For this review, take the finished solid that the model builds, in its own axes (mm). Face numbers are marked on the shaded views. A direction names the side the tool comes from. Round coordinates to 2 decimals unless told otherwise and drop trailing zeros. Order: outer loops, then holes, each group sorted by start corner. A loop starts at its lowest first (then second) coordinate and runs counter-clockwise, first axis right, second up.
from build123d import *
from OCP.BRepFilletAPI import BRepFilletAPI_MakeChamfer

# Parameters (mm, degrees)
SKETCH1_W           = 10.16
SKETCH1_H           = 25.4
BOSS_EXTRUDE1_DEPTH = 10.16
CHAMFER1_SIZE       = 5.08
CHAMFER1_SIZE2      = 3.557054294
CHAMFER6_SIZE       = 22.86
CHAMFER6_SIZE2      = 3.212763481
CHAMFER7_SIZE       = 22.86
CHAMFER7_SIZE2      = 3.212763481
CHAMFER10_SIZE2     = 1.466469684
CHAMFER10_SIZE      = 2.54
CHAMFER11_SIZE2     = 2.54
CHAMFER11_SIZE      = 1.466469684
BOSS_EXTRUDE2_DEPTH = 11.43
CHAMFER12_SIZE      = 20.32
CHAMFER12_SIZE_2    = 1.777769643
CHAMFER13_SIZE      = 1.27
CHAMFER13_SIZE2     = 0.703075315
CHAMFER13_SIZE2_2   = 0.738460687
CHAMFER14_SIZE      = 1.27
CHAMFER14_SIZE2     = 0.703075315
CHAMFER14_SIZE2_2   = 0.738460687
CHAMFER15_SIZE      = 29.032332849
CHAMFER15_SIZE_2    = 2.54
SCALE1_SCALE        = 1.5
BOSS_EXTRUDE4_DEPTH = 0.254


# Some blends are built 0.0001 mm under size
with BuildPart() as part:
    # Sketch1 → Boss-Extrude1 (new body)
    with BuildSketch(Plane.XY):
        with Locations((5.08, 12.7)):
            Rectangle(SKETCH1_W, SKETCH1_H)
    extrude(amount=BOSS_EXTRUDE1_DEPTH)

    # Chamfer1
    chamfer1_edges = [part.edges().sort_by_distance(p)[0] for p in [
        (5.08, 25.4, 10.16),
    ]]
    chamfer1_side = [part.faces().sort_by_distance(p)[0] for p in [
        (5.08, 12.7, 10.16),
    ]]
    chamfer(chamfer1_edges, length=CHAMFER1_SIZE, length2=CHAMFER1_SIZE2, reference=chamfer1_side[0])

    # Chamfer6
    chamfer6_edges = [part.edges().sort_by_distance(p)[0] for p in [
        (0, 0, 5.08),
    ]]
    chamfer6_side = [part.faces().sort_by_distance(p)[0] for p in [
        (0, 12.300671821, 4.93871201),
    ]]
    chamfer(chamfer6_edges, length=CHAMFER6_SIZE, length2=CHAMFER6_SIZE2, reference=chamfer6_side[0])

    # Chamfer7
    chamfer7_edges = [part.edges().sort_by_distance(p)[0] for p in [
        (10.16, 0, 5.08),
    ]]
    chamfer7_side = [part.faces().sort_by_distance(p)[0] for p in [
        (10.16, 12.300671821, 4.93871201),
    ]]
    chamfer(chamfer7_edges, length=CHAMFER7_SIZE, length2=CHAMFER7_SIZE2, reference=chamfer7_side[0])

    # Chamfer10
    chamfer10_edges = [part.edges().sort_by_distance(p)[0] for p in [
        (0, 25.4, 3.301472853),
    ]]
    chamfer10_side = [part.faces().sort_by_distance(p)[0] for p in [
        (0, 25.370670606, 3.301472853),
    ]]
    chamfer(chamfer10_edges, length=CHAMFER10_SIZE - 0.0001, length2=CHAMFER10_SIZE2 - 0.0001, reference=chamfer10_side[0])  # a hair under: the kernel refuses the full size

    # Chamfer11
    chamfer11_edges = [part.edges().sort_by_distance(p)[0] for p in [
        (10.16, 25.4, 3.301472853),
    ]]
    chamfer11_side = [part.faces().sort_by_distance(p)[0] for p in [
        (10.130670606, 25.4, 3.301472853),
    ]]
    chamfer(chamfer11_edges, length=CHAMFER11_SIZE - 0.0001, length2=CHAMFER11_SIZE2 - 0.0001, reference=chamfer11_side[0])  # a hair under: the kernel refuses the full size

    # Sketch2 → Boss-Extrude2 (add)
    with BuildSketch(Plane(origin=(0, 0, 0), x_dir=(-1, 0, 0), z_dir=(0, 0, -1))):
        Polygon((-5.08, 22.86), (-3.81, 22.86), (-3.81, 12.7), (-5.08, 12.7), (-6.35, 12.7), (-6.35, 22.86), align=None)
    extrude(amount=-BOSS_EXTRUDE2_DEPTH)

    # Chamfer12
    # the kernel refuses this chamfer: 20.32, 1.777769643 mm, written as the material it takes off along each edge
    with BuildSketch(Plane(origin=(-49.611801021, 0, 10.16), x_dir=(0, 0.9999943799678764, 0.003352615794033212), z_dir=(1, 0, 0))) as chamfer12_piece_1_section:
        Polygon((CHAMFER12_SIZE * 0.999994379968, -CHAMFER12_SIZE * 0.00335261579403), (-CHAMFER12_SIZE_2 * 0.00335261579374, -CHAMFER12_SIZE_2 * 0.999994379882), (0, 0), align=None)
    chamfer12_piece_1 = extrude(amount=109.383602042, mode=Mode.PRIVATE)
    chamfer12_piece_1 = split(chamfer12_piece_1, bisect_by=Plane(origin=(3.81, 16.274065634, 10.201831789), z_dir=(-1, 0, 0)), keep=Keep.TOP, mode=Mode.PRIVATE)
    chamfer12_piece_1 = split(chamfer12_piece_1, bisect_by=Plane(origin=(-22.90090051, 12.7, 10.201831789), z_dir=(0, 1, 0)), keep=Keep.TOP, mode=Mode.PRIVATE)
    add(chamfer12_piece_1, mode=Mode.SUBTRACT)
    with BuildSketch(Plane(origin=(-49.611801021, 0, 10.16), x_dir=(0, 0.9999943799678764, 0.003352615794033212), z_dir=(1, 0, 0))) as chamfer12_piece_2_section:
        Polygon((CHAMFER12_SIZE * 0.999994379968, -CHAMFER12_SIZE * 0.00335261579403), (-CHAMFER12_SIZE_2 * 0.00335261579374, -CHAMFER12_SIZE_2 * 0.999994379882), (0, 0), align=None)
    chamfer12_piece_2 = extrude(amount=109.383602042, mode=Mode.PRIVATE)
    chamfer12_piece_2 = split(chamfer12_piece_2, bisect_by=Plane(origin=(3.81, 5.349834898, 9.691469829), z_dir=(-1, 0, 0)), keep=Keep.TOP, mode=Mode.PRIVATE)
    chamfer12_piece_2 = split(chamfer12_piece_2, bisect_by=Plane(origin=(-22.90090051, 12.7, 9.691469829), z_dir=(0, -1, 0)), keep=Keep.TOP, mode=Mode.PRIVATE)
    add(chamfer12_piece_2, mode=Mode.SUBTRACT)
    with BuildSketch(Plane(origin=(-49.611801021, 0, 10.16), x_dir=(0, 0.9999943799678764, 0.003352615794033212), z_dir=(1, 0, 0))) as chamfer12_piece_3_section:
        Polygon((CHAMFER12_SIZE * 0.999994379968, -CHAMFER12_SIZE * 0.00335261579403), (-CHAMFER12_SIZE_2 * 0.00335261579374, -CHAMFER12_SIZE_2 * 0.999994379882), (0, 0), align=None)
    chamfer12_piece_3 = extrude(amount=109.383602042, mode=Mode.PRIVATE)
    chamfer12_piece_3 = split(chamfer12_piece_3, bisect_by=Plane(origin=(3.81, 5.349834898, 9.691469829), z_dir=(1, 0, 0)), keep=Keep.TOP, mode=Mode.PRIVATE)
    chamfer12_piece_3 = split(chamfer12_piece_3, bisect_by=Plane(origin=(5.08, 12.7, 9.691469829), z_dir=(0, -1, 0)), keep=Keep.TOP, mode=Mode.PRIVATE)
    chamfer12_piece_3 = split(chamfer12_piece_3, bisect_by=Plane(origin=(6.35, 5.349834898, 9.691469829), z_dir=(-1, 0, 0)), keep=Keep.TOP, mode=Mode.PRIVATE)
    add(chamfer12_piece_3, mode=Mode.SUBTRACT)
    with BuildSketch(Plane(origin=(-49.611801021, 0, 10.16), x_dir=(0, 0.9999943799678764, 0.003352615794033212), z_dir=(1, 0, 0))) as chamfer12_piece_4_section:
        Polygon((CHAMFER12_SIZE * 0.999994379968, -CHAMFER12_SIZE * 0.00335261579403), (-CHAMFER12_SIZE_2 * 0.00335261579374, -CHAMFER12_SIZE_2 * 0.999994379882), (0, 0), align=None)
    chamfer12_piece_4 = extrude(amount=109.383602042, mode=Mode.PRIVATE)
    chamfer12_piece_4 = split(chamfer12_piece_4, bisect_by=Plane(origin=(33.06090051, 12.7, 10.201831789), z_dir=(0, 1, 0)), keep=Keep.TOP, mode=Mode.PRIVATE)
    chamfer12_piece_4 = split(chamfer12_piece_4, bisect_by=Plane(origin=(6.35, 16.274065634, 10.201831789), z_dir=(1, 0, 0)), keep=Keep.TOP, mode=Mode.PRIVATE)
    add(chamfer12_piece_4, mode=Mode.SUBTRACT)
    with BuildSketch(Plane(origin=(-49.611801021, 0, 10.16), x_dir=(0, 0.9999943799678764, 0.003352615794033212), z_dir=(1, 0, 0))) as chamfer12_piece_5_section:
        Polygon((CHAMFER12_SIZE * 0.999994379968, -CHAMFER12_SIZE * 0.00335261579403), (-CHAMFER12_SIZE_2 * 0.00335261579374, -CHAMFER12_SIZE_2 * 0.999994379882), (0, 0), align=None)
    chamfer12_piece_5 = extrude(amount=109.383602042, mode=Mode.PRIVATE)
    chamfer12_piece_5 = split(chamfer12_piece_5, bisect_by=Plane(origin=(33.06090051, 12.7, 9.691469829), z_dir=(0, -1, 0)), keep=Keep.TOP, mode=Mode.PRIVATE)
    chamfer12_piece_5 = split(chamfer12_piece_5, bisect_by=Plane(origin=(6.35, 5.349834898, 9.691469829), z_dir=(1, 0, 0)), keep=Keep.TOP, mode=Mode.PRIVATE)
    add(chamfer12_piece_5, mode=Mode.SUBTRACT)

    # Chamfer13: one chamfer whose edges measure the first distance from different faces: ONE call of the kernel's chamfer builder (chamfer() names one face for all edges)
    chamfer13_edges_1 = [part.edges().sort_by_distance(p)[0] for p in [
        (0.17848686, 21.59, 9.270736426),
    ]]
    chamfer13_side_1 = [part.faces().sort_by_distance(p)[0] for p in [
        (5.08, 22.944432903, 8.322352298),
    ]]
    chamfer13_edges_2 = [part.edges().sort_by_distance(p)[0] for p in [
        (1.784868601, 10.16, 9.271115179),
    ]]
    chamfer13_side_2 = [part.faces().sort_by_distance(p)[0] for p in [
        (1.566458565, 11.714068156, 4.649741863),
    ]]
    chamfer13 = BRepFilletAPI_MakeChamfer(part.part.solid().wrapped)
    for e in chamfer13_edges_1:
        chamfer13.Add(CHAMFER13_SIZE, CHAMFER13_SIZE2, e.wrapped, chamfer13_side_1[0].wrapped)  # the first distance lies on this face
    for e in chamfer13_edges_2:
        chamfer13.Add(CHAMFER13_SIZE, CHAMFER13_SIZE2_2, e.wrapped, chamfer13_side_2[0].wrapped)  # the first distance lies on this face
    add(Compound.cast(chamfer13.Shape()), mode=Mode.REPLACE)

    # Chamfer14: one chamfer whose edges measure the first distance from different faces: ONE call of the kernel's chamfer builder (chamfer() names one face for all edges)
    chamfer14_edges_1 = [part.edges().sort_by_distance(p)[0] for p in [
        (9.98151314, 21.59, 9.270736426),
    ]]
    chamfer14_side_1 = [part.faces().sort_by_distance(p)[0] for p in [
        (8.593541435, 11.714068156, 4.649741863),
    ]]
    chamfer14_edges_2 = [part.edges().sort_by_distance(p)[0] for p in [
        (8.375131399, 10.16, 9.271115179),
    ]]
    chamfer14_side_2 = [part.faces().sort_by_distance(p)[0] for p in [
        (5.530551527, 10.889375046, 9.334927227),
    ]]
    chamfer14 = BRepFilletAPI_MakeChamfer(part.part.solid().wrapped)
    for e in chamfer14_edges_1:
        chamfer14.Add(CHAMFER14_SIZE, CHAMFER14_SIZE2, e.wrapped, chamfer14_side_1[0].wrapped)  # the first distance lies on this face
    for e in chamfer14_edges_2:
        chamfer14.Add(CHAMFER14_SIZE, CHAMFER14_SIZE2_2, e.wrapped, chamfer14_side_2[0].wrapped)  # the first distance lies on this face
    add(Compound.cast(chamfer14.Shape()), mode=Mode.REPLACE)

    # Chamfer15
    # the kernel refuses this chamfer: 29.032332849, 2.54 mm, written as the material it takes off along each edge
    with BuildSketch(Plane(origin=(-72.26067841, 0, 0), x_dir=(0, 0.9999943799678764, -0.0033526157940330635), z_dir=(1, 0, 0))) as chamfer15_piece_1:
        Polygon((CHAMFER15_SIZE * 0.999994379968, CHAMFER15_SIZE * 0.00335261579403), (-CHAMFER15_SIZE_2 * 0.00335261579403, CHAMFER15_SIZE_2 * 0.999994379968), (0, 0), align=None)
    extrude(amount=154.68135682, mode=Mode.SUBTRACT)


with BuildPart() as part_1:
    # Scale1: scaled about (5.081275253, 15.154751407, 5.333676916)
    add(part.part.scale(SCALE1_SCALE).moved(Location((-2.540637627, -7.577375703, -2.666838458))))


with BuildPart() as boss_extrude4_tool:
    # Sketch5 → Boss-Extrude4 (new body)
    with BuildSketch(Plane(origin=(0, 0.041695217, 0.476578517), x_dir=(-1, 0, 0), z_dir=(0, -0.08715574274765502, -0.9961946980917459))):
        Polygon((-8.031077325, 26.787369773), (-5.079362375, 26.787369773), (-2.127647425, 26.787369773), (-2.127647425, 17.698761839), (-8.031077325, 17.698761839), align=None)
    extrude(amount=BOSS_EXTRUDE4_DEPTH)


with BuildPart() as part_2:
    add(part_1.part)


with BuildPart() as part_3:
    # Boss-Extrude4: joined with boss_extrude4_tool
    add(part_2.part.fuse(boss_extrude4_tool.part, tol=0.00001))


solid = part_3.part
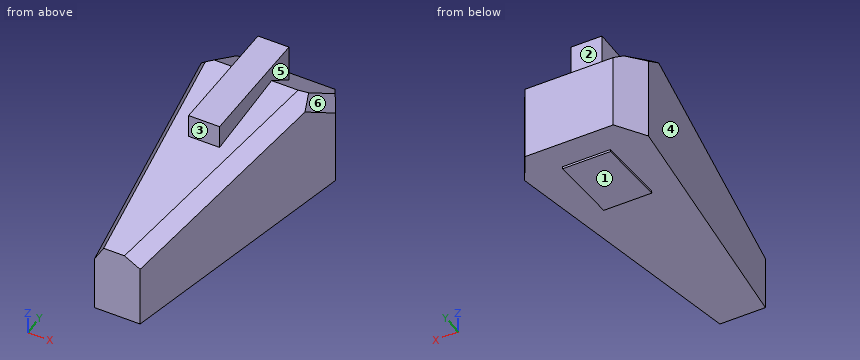
(1) Add section D-D on x = 7.5. Give the boundary of the cut face in (y, z) (3 decimals).
(2) Draft analysis for pull direction Y (two halves, no side actions). For the marked faces 4, 5 and 6, state which applies: pulls with the +Y half, pulls with the -Y half, needs draft (parallel to the pull), parting line crosses it, or undercut.
(3) Add section C-C on y = 0. Give the boundary of the cut face in (x, z), plus the area to 3 significant figures.
(4) Clearance check with flat-ended pins moving along their axes: P1, Ø2.5, axis at y = 22, z = 11.5, coming from the -X side; P2, Ø0.8, axis at y = 23.5, z = -1.5, coming from the -X side; P3, Ø3, axis at x = 5.5, z = 13, coming from the +Y side; P4, Ø6, axis at x = 3, z = 12, coming from the -Y side. State where each tip first meets the part, or that it passes through.
(5) Wall thickness on L1, parallel to X at y = 11, z = 7.75; L2, parallel to Y at x = 4.75, z = 12.75; L3, parallel to X at y = 17, z = -0.75: over which ranges is each line inside the solid? List them lowest first.
(6) Tool access review of the marked faces 1, 2 and 3: name each direction out of +Z, -Z, +X, -X, +Y, -Y from which nothing blocks a thin tool from reaching the whole face with its end or side.
Here are the results:
1. outline: (-7.577, 1.143) - (17.673, -1.066) - (17.651, -1.319) - (26.705, -2.111) - (26.727, -1.858) - (30.523, -2.19) - (30.523, 7.238) - (22.903, 12.573) - (3.404, 10.867) - (-7.577, 9.014) - close
2. face 4: pulls with the -Y half
2. face 5: needs draft
2. face 6: pulls with the +Y half
3. outline: (1.21, 0.48) - (8.95, 0.48) - (8.95, 9.46) - (7.02, 10.57) - (2.33, 10.57) - (1.21, 8.66) - close
3. area: 75.9 mm2
4. P1: stops at x = -2.01
4. P2: stops at x = -2.15
4. P3: stops at y = 26.71
4. P4: stops at y = -7.58
5. L1: x = -0.33 to 10.49
5. L2: y = 11.47 to 26.71
5. L3: x = -1.18 to 11.33
6. face 1: -Z, +X, -X, -Y
6. face 2: +Z, +X, -X, +Y
6. face 3: +Z, +X, -X, -Y
